from build123d import *

# Parameters (mm, degrees)
SKETCH1_W           = 500
SKETCH1_H           = 350
BOSS_EXTRUDE2_DEPTH = 140
SKETCH2_R           = 17.5
CUT_EXTRUDE1_DEPTH  = 10
SKETCH3_R           = 15
CUT_EXTRUDE2_DEPTH  = 10
SKETCH4_W           = 480
SKETCH4_H           = 330
CUT_EXTRUDE3_DEPTH  = 130
FILLET1_R           = 10
FILLET3_R           = 5


with BuildPart() as part:
    # Sketch1 → Boss-Extrude2 (new body)
    with BuildSketch(Plane.XY):
        Rectangle(SKETCH1_W, SKETCH1_H)
    extrude(amount=BOSS_EXTRUDE2_DEPTH)

    # Sketch2 → Cut-Extrude1 (cut)
    with BuildSketch(Plane(origin=(250, 0, 0), x_dir=(0, 0, -1), z_dir=(1, 0, 0))):
        with Locations(Location((-52.403317004, -94.104000371, 0), (0, 0, 90))):
            Circle(SKETCH2_R)
    extrude(amount=-CUT_EXTRUDE1_DEPTH, mode=Mode.SUBTRACT)

    # Sketch3 → Cut-Extrude2 (cut)
    with BuildSketch(Plane(origin=(0, 175, 0), x_dir=(1, 0, 0), z_dir=(0, 1, 0))):
        with Locations(Location((172.864228893, -58.246086874, 0), (0, 0, 270))):
            Circle(SKETCH3_R)
    extrude(amount=-CUT_EXTRUDE2_DEPTH, mode=Mode.SUBTRACT)

    # Sketch4 → Cut-Extrude3 (cut)
    with BuildSketch(Plane.XY.offset(140)):
        Rectangle(SKETCH4_W, SKETCH4_H)
    extrude(amount=-CUT_EXTRUDE3_DEPTH, mode=Mode.SUBTRACT)

    # Fillet1
    fillet1_edges = [part.edges().sort_by_distance(p)[0] for p in [
        (250, -175, 70),
        (-250, -175, 70),
        (-250, 175, 70),
        (250, 175, 70),
    ]]
    fillet(fillet1_edges, radius=FILLET1_R)

    # Fillet3
    fillet3_edges = [part.edges().sort_by_distance(p)[0] for p in [
        (0, 175, 0),
        (250, 0, 0),
        (0, -175, 0),
        (-250, 0, 0),
        (-247.071067812, -172.071067812, 0),
        (-247.071067812, 172.071067812, 0),
        (247.071067812, -172.071067812, 0),
        (247.071067812, 172.071067812, 0),
    ]]
    fillet(fillet3_edges, radius=FILLET3_R)


solid = part.part
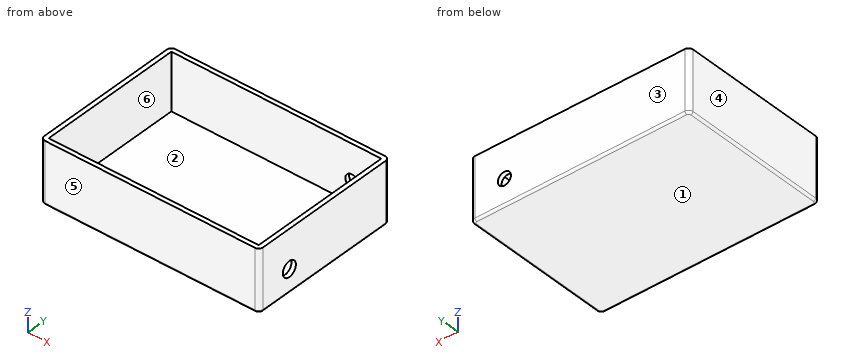
CAD build for the part. Positions are in the model's coordinates, mm. Face numbers are marked on the shaded views. A direction names the side the tool comes from. Give positions to 0.01 mm unless a question says otherwise; leave off trailing zeros. Write each loop counter-clockwise with the first axis right and the second up, starting at its lowest first coordinate (ties: lowest second). Pieces come first, ordered by that corner, then holes. Notation, with made-up numbers: M 1,70.25 L 21,70.25 A21 ccw 21,103.25 Z; hole C 64,-7 d4. An arc over 180 degrees is marked long. Put each result on its own line as item: value. Start each with the question number.
(1) Band-saw the part on B-B, the plane y = -128.5. Write the cut outline in (x, z), and give its area (3 significant figures).
(2) Band-saw the part on A-A, the plane z = 119. Write the cut outline in (x, y), and give its area (3 significant figures).
(3) Flat gauge pin, fed straight in: pin 1 Ø6 at (x, y) = (-144.5, -89.5) entering from +Z. Where does the tip first touch, or does it go through?
(4) Mould opens along Y. For the marked faces 3, 4, 5 and 6 say: +Y half, -Y half, draft (parallel to the pull), parting line (faces both ways), or undercut.
(5) Band-saw the part on C-C, the plane z = 63.5. Write the cut outline in (x, y), and give its area (3 significant figures).
(6) Probe L1, parallel to X at y = 27, z = 55; L2, parallel to Y at x = 128, z = 71.5; L3, parallel to Z at x = 93.5, y = -64. List the from-to ranges inside material, lowest first.
(7) Which spindle directions (+Z, -Z, +X, -X, +Y, -Y) get a long thin tool onto all of the face, cutting with end or side? Do the marked faces 1 and 2. Say none if no direction does.
(8) Band-saw the part on D-D, the plane x = -10. Write the cut outline in (y, z), and give its area (3 significant figures).
Response values:
1. outline: M -250,5 A5 ccw -245,0 L 245,0 A5 ccw 250,5 L 250,140 L 240,140 L 240,10 L -240,10 L -240,140 L -250,140 Z
1. area: 7,590 mm2
2. outline: M -250,-165 A10 ccw -240,-175 L 240,-175 A10 ccw 250,-165 L 250,165 A10 ccw 240,175 L -240,175 A10 ccw -250,165 Z; hole M -240,-165 L 240,-165 L 240,165 L -240,165 Z
2. area: 16,500 mm2
3. pin 1: stops at z = 10
4. face 3: +Y half
4. face 4: draft
4. face 5: -Y half
4. face 6: undercut
5. outline: M -250,-165 A10 ccw -240,-175 L 240,-175 A10 ccw 250,-165 L 250,-107.64 L 240,-107.64 L 240,-165 L -240,-165 L -240,165 L 158.81,165 L 158.81,175 L -240,175 A10 ccw -250,165 Z; M 186.91,165 L 240,165 L 240,-80.57 L 250,-80.57 L 250,165 A10 ccw 240,175 L 186.91,175 Z
5. area: 16,000 mm2
6. L1: x = -250 to -240, 240 to 250
6. L2: y = -175 to -165, 165 to 175
6. L3: z = 0 to 10
7. face 1: -Z, +X, -X, +Y, -Y
7. face 2: +Z
8. outline: M -175,5 A5 ccw -170,0 L 170,0 A5 ccw 175,5 L 175,140 L 165,140 L 165,10 L -165,10 L -165,140 L -175,140 Z
8. area: 6,090 mm2
